```python
from build123d import *

# Parameters (mm, degrees)
F0_W      = 5
F0_H      = 5
F1_DEPTH  = 90
F2_W      = 5
F2_H      = 5
F3_DEPTH  = 90
F4_W      = 5
F4_H      = 5
F5_DEPTH  = 90
F6_W      = 5
F6_H      = 5
F7_DEPTH  = 90
F8_W      = 5
F8_H      = 5
F9_DEPTH  = 90
F10_R     = 2.5
F11_DEPTH = 35
F12_W     = 5
F12_H     = 5
F13_DEPTH = 85
F14_W     = 5
F14_H     = 4
F15_DEPTH = 0.3
F16_R     = 0.8
F17_DEPTH = 0.3
F18_W     = 2.5
F18_H     = 2.5
F18_W_2   = 2
F18_H_2   = 2
F19_DEPTH = 0.3
F20_R     = 0.8
F21_DEPTH = 0.3
F22_W     = 2.5
F22_H     = 2.5
F22_W_2   = 2
F22_H_2   = 2
F23_DEPTH = 0.3


with BuildPart() as f1:
    # F0 (on Front) → F1 (new body)
    with BuildSketch(Plane.XZ):
        Rectangle(F0_W, F0_H)
    extrude(amount=-F1_DEPTH)

    # F2 (on face) → F3 (join)
    with BuildSketch(Plane(origin=(-2.5, 0, 0), x_dir=(0, -1, 0), z_dir=(-1, 0, 0))):
        with Locations((-87.5, 0)):
            Rectangle(F2_W, F2_H)
    extrude(amount=F3_DEPTH)

    # F4 (on face) → F5 (join)
    with BuildSketch(Plane.XZ.offset(-85)):
        with Locations((-90, 0)):
            Rectangle(F4_W, F4_H)
    extrude(amount=F5_DEPTH)

    # F6 (on face) → F7 (join)
    with BuildSketch(Plane.YZ.offset(-87.5)):
        with Locations((-2.5, 0)):
            Rectangle(F6_W, F6_H)
    extrude(amount=F7_DEPTH)

    # F8 (on face) → F9 (join)
    with BuildSketch(Plane.YZ.offset(-87.5)):
        with Locations((70.5, 0)):
            Rectangle(F8_W, F8_H)
    extrude(amount=F9_DEPTH)

    # F10 (on face) → F11 (join)
    with BuildSketch(Plane.XZ.offset(-68)):
        with Locations((-45, 0)):
            Circle(F10_R)
    extrude(amount=F11_DEPTH)

    # F12 (on face) → F13 (join)
    with BuildSketch(Plane.YZ.offset(-87.5)):
        with Locations((30.5, 0)):
            Rectangle(F12_W, F12_H)
    extrude(amount=F13_DEPTH)

    # F14 (on face) → F15 (cut)
    with BuildSketch(Plane(origin=(0, 0, -2.5), x_dir=(1, 0, 0), z_dir=(0, 0, -1))):
        with Locations((-65, -30.5)):
            Rectangle(F14_W, F14_H)
        with Locations((-25, -30.5)):
            Rectangle(F14_W, F14_H)
    extrude(amount=-F15_DEPTH, mode=Mode.SUBTRACT)

    # F16 (on face) → F17 (join)
    with BuildSketch(Plane(origin=(0, 0, -2.2), x_dir=(1, 0, 0), z_dir=(0, 0, -1))):
        with Locations((-65, -30.5)):
            Circle(F16_R)
    extrude(amount=F17_DEPTH)

    # F18 (on face) → F19 (cut)
    with BuildSketch(Plane(origin=(0, 0, -2.2), x_dir=(1, 0, 0), z_dir=(0, 0, -1))):
        with Locations((-65, -30.5)):
            Rectangle(F18_W, F18_H)
        with Locations((-65, -30.5)):
            Rectangle(F18_W_2, F18_H_2, mode=Mode.SUBTRACT)
    extrude(amount=-F19_DEPTH, mode=Mode.SUBTRACT)

    # F20 (on face) → F21 (join)
    with BuildSketch(Plane(origin=(0, 0, -2.2), x_dir=(1, 0, 0), z_dir=(0, 0, -1))):
        with Locations((-25, -30.5)):
            Circle(F20_R)
    extrude(amount=F21_DEPTH)

    # F22 (on face) → F23 (cut)
    with BuildSketch(Plane(origin=(0, 0, -2.2), x_dir=(1, 0, 0), z_dir=(0, 0, -1))):
        with Locations((-25, -30.5)):
            Rectangle(F22_W, F22_H)
        with Locations((-25, -30.5)):
            Rectangle(F22_W_2, F22_H_2, mode=Mode.SUBTRACT)
    extrude(amount=-F23_DEPTH, mode=Mode.SUBTRACT)


solid = f1.part
```
Input: part model. Units: mm. Frame: model coordinates. A direction names the side the tool comes from. Coordinates: 2 decimals unless noted, no trailing zeros. Loops run counter-clockwise (first coordinate to the right, second up) from the corner with the lowest first, then second, coordinate; pieces in that order, holes last. Notation, with made-up numbers: (-7, 78) - (17, 78) arc R16 ccw to (17, 85) - close; hole circle Ø3 at (35, -36.5). An arc over 180 degrees is marked (long way). Answer in a Markdown table with one row per item.
(1) Cut plane D-D on z = 0. Output: boundary loops of the cut face in (x, y).
Model answer:
| item | result |
|---|---|
| outline | (-92.5, -5) - (2.5, -5) - (2.5, 90) - (-92.5, 90) - close; hole (-87.5, 0) - (-2.5, 0) - (-2.5, 28) - (-87.5, 28) - close; hole (-87.5, 33) - (-47.5, 33) - (-47.5, 68) - (-87.5, 68) - close; hole (-87.5, 73) - (-2.5, 73) - (-2.5, 85) - (-87.5, 85) - close; hole (-42.5, 33) - (-2.5, 33) - (-2.5, 68) - (-42.5, 68) - close |
(2) Cut plane B-B on x = -82.5. Output: boundary loops of the cut face in (y, z), plus the area to 3 significant figures.
Model answer:
| item | result |
|---|---|
| outline | (-5, -2.5) - (0, -2.5) - (0, 2.5) - (-5, 2.5) - close; (28, -2.5) - (33, -2.5) - (33, 2.5) - (28, 2.5) - close; (68, -2.5) - (73, -2.5) - (73, 2.5) - (68, 2.5) - close; (85, -2.5) - (90, -2.5) - (90, 2.5) - (85, 2.5) - close |
| area | 100 mm² |
(3) Material intervals for L1, parallel to Y at x = -24.5, z = 0.2; L2, parallel to Y at x = -44, z = 1.05; L3, parallel to X at y = 13, z = 1.3, sorted ascending. Write a range as from..to.
Model answer:
| item | result |
|---|---|
| L1 | y = -5..0, 28..33, 68..73, 85..90 |
| L2 | y = -5..0, 28..73, 85..90 |
| L3 | x = -92.5..-87.5, -2.5..2.5 |
(4) Cut plane A-A on y = 76.5. Output: boundary loops of the cut face in (x, z).
Model answer:
| item | result |
|---|---|
| outline | (-92.5, -2.5) - (-87.5, -2.5) - (-87.5, 2.5) - (-92.5, 2.5) - close; (-2.5, -2.5) - (2.5, -2.5) - (2.5, 2.5) - (-2.5, 2.5) - close |
(5) Set-up query: faces 1 (the face through (-42.69, 50.74, -0.96)), 2 (the face through (-87.5, 14, 0)), 3 (the face through (-92.5, 43, 0)). Return all of +Z, -Z, +X, -X, +Y, -Y with unobstructed straight access to the full face (end or side cutting, diameter ignored); none if empty.
Model answer:
| item | result |
|---|---|
| face 1 | none |
| face 2 | +Z, -Z |
| face 3 | +Z, -Z, -X, +Y, -Y |
(6) Mould query, pull axis Y, two halves, no side actions, for faces 4 (the face through (2.5, 42, 0)), 5 (the face through (-2.5, 50, 0)). Classes: pulls with the +Y half, pulls with the -Y half, needs draft (parallel to the pull), parting line crosses it, or undercut.
Model answer:
| item | result |
|---|---|
| face 4 | needs draft |
| face 5 | undercut |
(7) Cut plane C-C on y = 38. Output: boundary loops of the cut face in (x, z), plus the area to 3 significant figures.
Model answer:
| item | result |
|---|---|
| outline | (-92.5, -2.5) - (-87.5, -2.5) - (-87.5, 2.5) - (-92.5, 2.5) - close; circle Ø5 at (-45, 0); (-2.5, -2.5) - (2.5, -2.5) - (2.5, 2.5) - (-2.5, 2.5) - close |
| area | 69.6 mm² |
